For this review, use the dimensioned drawing (mm, ordinates from the lowest corner) and the shaded views. A direction names the side the tool comes from. Give positions to 0.01 mm unless a question says otherwise; leave off trailing zeros. Order: outer loops, then holes, each group sorted by start corner. A loop starts at its lowest first (then second) coordinate and runs counter-clockwise, first axis right, second up. Notation, with made-up numbers: (-27, 32.25) - (-5, 32.25) arc R15 ccw to (-5, 43.25) - close; hole circle Ø7 at (-21, -30.5). An arc over 180 degrees is marked (long way). One line per item, written item: value.
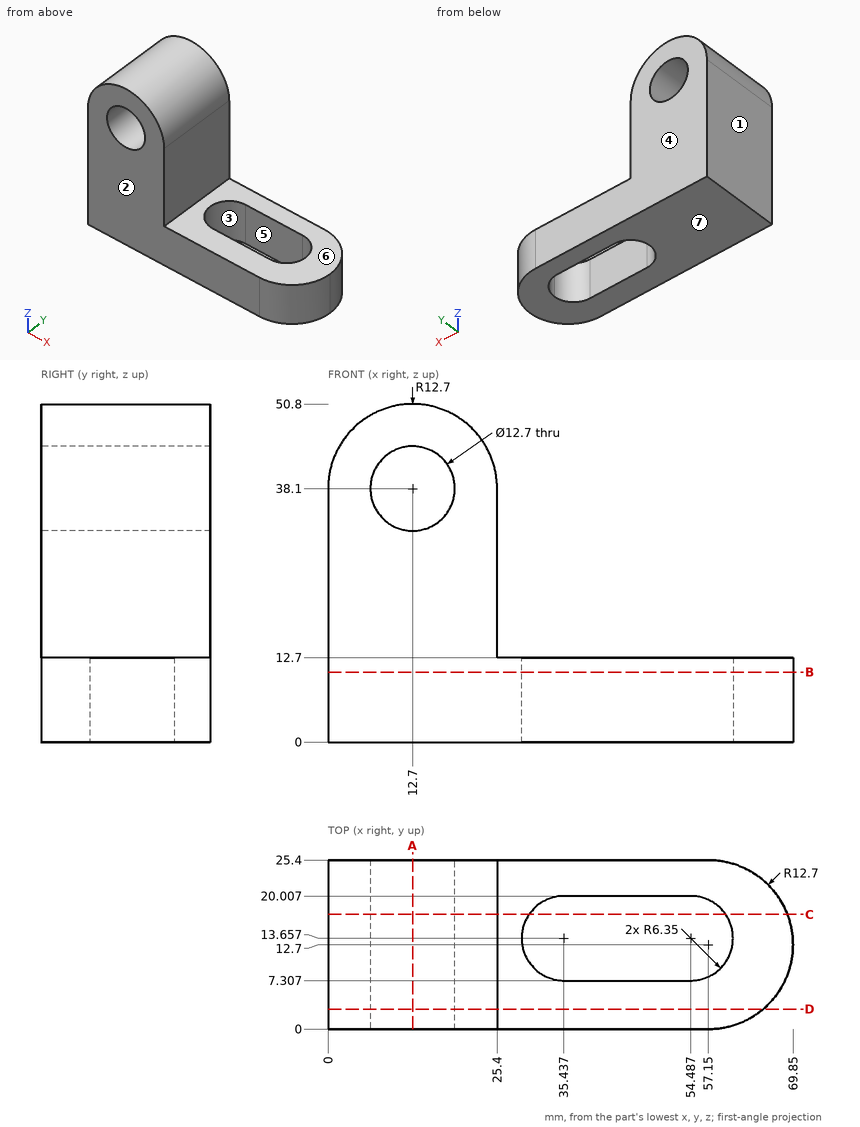
(1) Take a section at A-A (x = 12.7). Write out the cut boundary in (y, z).
Answers below:
outline: (0, 0) - (25.4, 0) - (25.4, 31.75) - (0, 31.75) - close; (0, 44.45) - (25.4, 44.45) - (25.4, 50.8) - (0, 50.8) - close
(2) Draft analysis for pull direction Y (two halves, no side actions). For the marked faces 1, 2, 3 and 4, state which applies: pulls with the +Y half, pulls with the -Y half, needs draft (parallel to the pull), parting line crosses it, or undercut.
Answers below:
face 1: needs draft
face 2: pulls with the -Y half
face 3: undercut
face 4: pulls with the +Y half
(3) Wall thickness on line 1 (Z direction, x = 12.7, y = 9); line 2 (X direction, y = 14, z = 24); line 3 (Z direction, x = 46.5, y = 22.5): over which ranges is each line inside the solid? List them lowest first. Write a range as from..to.
Answers below:
line 1: z = 0..31.75, 44.45..50.8
line 2: x = 0..25.4
line 3: z = 0..12.7
(4) Take a section at B-B (z = 10.5). Write out the cut boundary in (x, y), then the cut area to 3 significant figures.
Answers below:
outline: (0, 0) - (57.15, 0) arc R12.7 ccw to (57.15, 25.4) - (0, 25.4) - close; hole (35.44, 7.31) - (54.49, 7.31) arc R6.35 ccw to (54.49, 20.01) - (35.44, 20.01) arc R6.35 ccw to start
area: 1,340 mm^2
(5) For P1, Ø10, axis at x = 47, z = 8.5, coming from the -Y side; P2, Ø6, axis at y = 15, z = 35.5, coming from the +X side; P3, Ø10, axis at x = 19.5, y = 20.5, coming from the +Z side; P4, Ø10, axis at x = 21, y = 14.5, coming from the +Z side, all flat-tipped, find the tip position at first contact; note any pin that passes through.
Answers below:
P1: stops at y = 0
P2: stops at x = 25.4
P3: stops at z = 50.67
P4: stops at z = 50.36
(6) Take a section at C-C (y = 17.25). Write out the cut boundary in (x, z).
Answers below:
outline: (0, 0) - (30.2, 0) - (30.2, 12.7) - (25.4, 12.7) - (25.4, 38.1) arc R12.7 ccw to (0, 38.1) - close; (59.72, 0) - (69.01, 0) - (69.01, 12.7) - (59.72, 12.7) - close; hole circle Ø12.7 at (12.7, 38.1)
(7) Machinability: for the marked faces 5, 6 and 7, which of the approach directions +Z, -Z, +X, -X, +Y, -Y give a long, thin tool a straight path to every point of the face, cutting with its end or side? Answer none if there is none.
Answers below:
face 5: +Z, -Z
face 6: +Z, +X, +Y, -Y
face 7: -Z, +X, -X, +Y, -Y
(8) Take a section at D-D (y = 3). Write out the cut boundary in (x, z), then the cut area to 3 significant figures.
Answers below:
outline: (0, 0) - (65.35, 0) - (65.35, 12.7) - (25.4, 12.7) - (25.4, 38.1) arc R12.7 ccw to (0, 38.1) - close; hole circle Ø12.7 at (12.7, 38.1)
area: 1,600 mm^2
